```python
from build123d import *

# Parameters (mm, degrees)
CYLINDER050_R     = 22.5
CYLINDER050_DEPTH = 28
CYLINDER049_R     = 43
CYLINDER049_DEPTH = 28
FILLET_R          = 2
CHAMFER_SIZE      = 4
FILLET010_R       = 3


with BuildPart() as cylinder050:
    # Cylinder050 → Cylinder050 (new body)
    with BuildSketch(Plane.XZ):
        Circle(CYLINDER050_R)
    extrude(amount=CYLINDER050_DEPTH)


with BuildPart() as wheel_wide_left:
    # Cylinder049 → Cylinder049 (new body)
    with BuildSketch(Plane.XZ):
        Circle(CYLINDER049_R)
    extrude(amount=CYLINDER049_DEPTH)

    # Cut019: cut Cylinder050
    add(cylinder050.part, mode=Mode.SUBTRACT)

    # Fillet
    fillet_edges = [wheel_wide_left.edges().sort_by_distance(p)[0] for p in [
        (-43, -28, 0),
        (-43, 0, 0),
    ]]
    fillet(fillet_edges, radius=FILLET_R)

    # Chamfer
    chamfer_edges = [wheel_wide_left.edges().sort_by_distance(p)[0] for p in [
        (-22.5, 0, 0),
        (-22.5, -28, 0),
    ]]
    chamfer(chamfer_edges, length=CHAMFER_SIZE)

    # Fillet010
    fillet010_edges = [wheel_wide_left.edges().sort_by_distance(p)[0] for p in [
        (-26.5, 0, 0),
        (-26.5, -28, 0),
    ]]
    fillet(fillet010_edges, radius=FILLET010_R)


with BuildPart() as wheel_wide_left_1:
    # Fillet010 placement: moved
    add(wheel_wide_left.part.moved(Location((0, -63, 0))))


solid = wheel_wide_left_1.part
```
Geometry: final body of the model. Coordinates: model frame, mm. Coordinates: 2 decimals unless noted, no trailing zeros. Order: outer loops, then holes, each group sorted by start corner. A loop starts at its lowest first (then second) coordinate and runs counter-clockwise, first axis right, second up. Notation, with made-up numbers: (-8, 58) -> (14, 58) arc R21 cw to (14, 84) -> close; hole circle Ø8 at (-6, 87). An arc over 180 degrees is marked (long way). Write item = value, one per line.
(1) Cut plane A-A on z = 0. Return loops of the section in (x, y).
Solved:
outline = (-43, -89) arc R2 ccw to (-41, -91) -> (-27.74, -91) arc R3 ccw to (-25.62, -90.12) -> (-22.5, -87) -> (-22.5, -67) -> (-25.62, -63.88) arc R3 ccw to (-27.74, -63) -> (-41, -63) arc R2 ccw to (-43, -65) -> close; (22.5, -87) -> (25.62, -90.12) arc R3 ccw to (27.74, -91) -> (41, -91) arc R2 ccw to (43, -89) -> (43, -65) arc R2 ccw to (41, -63) -> (27.74, -63) arc R3 ccw to (25.62, -63.88) -> (22.5, -67) -> close
(2) Line query: line 1 (Z direction, x = 0, y = -71); line 2 (X direction, y = -72.75, z = 13); line 3 (X direction, y = -87.5, z = 6). Output: solid intervals per line, ascending.
Solved:
line_1 = -43 to -22.5, 22.5 to 43
line_2 = -40.99 to -18.36, 18.36 to 40.99
line_3 = -42.58 to -22.2, 22.2 to 42.58
(3) Cut plane C-C on y = -82.5. Return loops of the section in (x, z).
Solved:
outline = circle Ø86 at (0, 0); hole circle Ø45 at (0, 0)
(4) Pin query (flat end, axial travel): pin 1 Ø4 at (x, y) = (-10.5, -77) entering from -Z; pin 2 Ø10 at (y, z) = (-67.5, 13.5) entering from -X; pin 3 Ø5 at (x, y) = (-19, -67.5) entering from +Z. Return the tip coordinate at first contact, or that it passes through.
Solved:
pin_1 = -42.15
pin_2 = -42.15
pin_3 = 39.71
(5) Pull-direction query (Z, two-part tool) for faces 1 (the cylindrical face through (-5.598, -76.832, 42.634)), 2 (the cylindrical face through (10.382, -76.86, -19.961)), 3 (the conical face through (-4.91, -66.85, -22.11)), 4 (the flat face through (27, -63, -9)); classes: pulls with the +Z half, pulls with the -Z half, needs draft (parallel to the pull), parting line crosses it, or undercut.
Solved:
face_1 = parting line crosses it
face_2 = undercut
face_3 = undercut
face_4 = needs draft
(6) Cut plane B-B on x = 0. Return loops of the section in (y, z), plus the area to 3 significant figures.
Solved:
outline = (-91, -41) arc R2 ccw to (-89, -43) -> (-65, -43) arc R2 ccw to (-63, -41) -> (-63, -27.74) arc R3 ccw to (-63.88, -25.62) -> (-67, -22.5) -> (-87, -22.5) -> (-90.12, -25.62) arc R3 ccw to (-91, -27.74) -> close; (-91, 27.74) arc R3 ccw to (-90.12, 25.62) -> (-87, 22.5) -> (-67, 22.5) -> (-63.88, 25.62) arc R3 ccw to (-63, 27.74) -> (-63, 41) arc R2 ccw to (-65, 43) -> (-89, 43) arc R2 ccw to (-91, 41) -> close
area = 1,110 mm²
